from build123d import *

# Parameters (mm, degrees)
F0_W     = 40
F0_H     = 40
F0_R     = 2.15
F0_R_2   = 19.5
F1_DEPTH = 10
F2_R     = 3


with BuildPart() as f1:
    # F0 (on Top) → F1 (new body)
    with BuildSketch(Plane.XY):
        with Locations((-20, 20)):
            Rectangle(F0_W, F0_H)
        with Locations((-36, 4)):
            Circle(F0_R, mode=Mode.SUBTRACT)
        with Locations((-4, 4)):
            Circle(F0_R, mode=Mode.SUBTRACT)
        with Locations((-36, 36)):
            Circle(F0_R, mode=Mode.SUBTRACT)
        with Locations((-20, 20)):
            Circle(F0_R_2, mode=Mode.SUBTRACT)
        with Locations((-4, 36)):
            Circle(F0_R, mode=Mode.SUBTRACT)
    extrude(amount=F1_DEPTH)

    # F2
    f2_edges = [f1.edges().sort_by_distance(p)[0] for p in [
        (0, 0, 5),
        (0, 40, 5),
        (-40, 40, 5),
        (-40, 0, 5),
    ]]
    fillet(f2_edges, radius=F2_R)


solid = f1.part
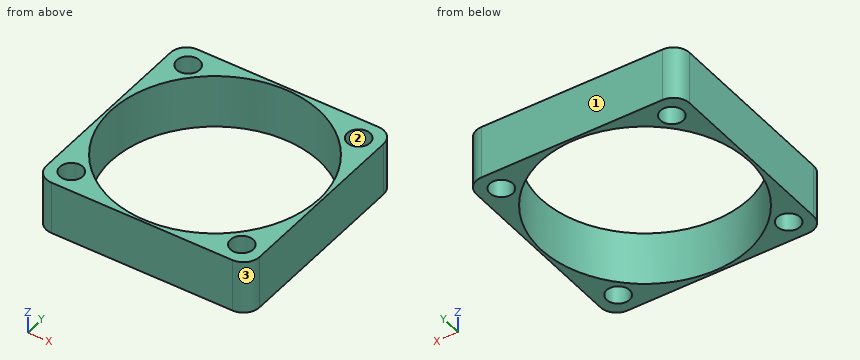
Source: CAD feature listing. Evaluate the final solid. Frame: model axes, mm. Face numbers are marked on the shaded views. Coordinates: 2 decimals unless noted, no trailing zeros. Loops run counter-clockwise (first coordinate to the right, second up) from the corner with the lowest first, then second, coordinate; pieces in that order, holes last. Notation, with made-up numbers: (26.5, 58) - (52.5, 58) arc R35 cw to (52.5, 96) - close; hole circle Ø5 at (-1, 61.25). An arc over 180 degrees is marked (long way). Return JSON: item names as keys, results as strings.
Q1. Mould query, pull axis X, two halves, no side actions, for the marked faces 1, 2 and 3. Classes: released by +X, released by -X, zero draft, split by the parting line, or undercut.
Results:
{"face 1": "zero draft", "face 2": "undercut", "face 3": "released by +X"}
Q2. Material intervals for line 1 along Y through (x, z) = (-4, 6.25); line 2 along Y through (x, z) = (-37.5, 7.75); line 3 along Y through (x, z) = (-20, 6.75), sorted ascending.
Results:
{"line 1": "0 to 1.85, 6.15 to 8.85, 31.15 to 33.85, 38.15 to 40", "line 2": "0.04 to 2.46, 5.54 to 11.4, 28.6 to 34.46, 37.54 to 39.96", "line 3": "0 to 0.5, 39.5 to 40"}
Q3. Section B-B, the plane z = 3. Return loops of the section in (x, y), plus the area to 3 significant figures.
Results:
{"outline": "(-40, 3) arc R3 ccw to (-37, 0) - (-3, 0) arc R3 ccw to (0, 3) - (0, 37) arc R3 ccw to (-3, 40) - (-37, 40) arc R3 ccw to (-40, 37) - close; hole circle Ø39 at (-20, 20); hole circle Ø4.3 at (-36, 4); hole circle Ø4.3 at (-36, 36); hole circle Ø4.3 at (-4, 4); hole circle Ø4.3 at (-4, 36)", "area": "340 mm2"}
Q4. Section C-C, the plane x = -20. Return loops of the section in (y, z), plus the area to 3 significant figures.
Results:
{"outline": "(0, 0) - (0.5, 0) - (0.5, 10) - (0, 10) - close; (39.5, 0) - (40, 0) - (40, 10) - (39.5, 10) - close", "area": "10.0 mm2"}
Q5. Section A-A, the plane y = 20. Return loops of the section in (x, z).
Results:
{"outline": "(-40, 0) - (-39.5, 0) - (-39.5, 10) - (-40, 10) - close; (-0.5, 0) - (0, 0) - (0, 10) - (-0.5, 10) - close"}
Q6. Section D-D, the plane x = -36.5. Return loops of the section in (y, z), plus the area to 3 significant figures.
Results:
{"outline": "(0, 0) - (1.91, 0) - (1.91, 10) - (0, 10) - close; (6.09, 0) - (9.61, 0) - (9.61, 10) - (6.09, 10) - close; (30.39, 0) - (33.91, 0) - (33.91, 10) - (30.39, 10) - close; (38.09, 0) - (40, 0) - (40, 10) - (38.09, 10) - close", "area": "109 mm2"}
